Design review of the part built by this model. Coordinates are the model's own, in mm. Face numbers are marked on the shaded views. A direction names the side the tool comes from. Give positions to 0.01 mm unless a question says otherwise; leave off trailing zeros. Order: outer loops, then holes, each group sorted by start corner. A loop starts at its lowest first (then second) coordinate and runs counter-clockwise, first axis right, second up. Notation, with made-up numbers: (13.25, 61.5) - (69.25, 61.5) arc R19 cw to (69.25, 97.5) - close; hole circle Ø5 at (74.5, 26). An arc over 180 degrees is marked (long way). Write each question's results on one line, items separated by ' | '. Start each with the question number.
```python
from build123d import *

# Parameters (mm, degrees)
SKETCH1_R           = 4.15
BOSS_EXTRUDE1_DEPTH = 10
SKETCH4_R           = 11
CUT_EXTRUDE2_DEPTH  = 7.2
CHAMFER1_SIZE       = 1
FILLET2_R           = 25
FILLET3_R           = 2
FILLET4_R           = 2
FILLET5_DEPTH       = 11
FILLET5_2_ANGLE     = 84.965742
FILLET5_3_ANGLE     = 84.965742
SKETCH5_R           = 2.8
CUT_EXTRUDE3_DEPTH  = 58.10630094
CUT_EXTRUDE5_DEPTH  = 4
SKETCH8_R           = 1.5
CUT_EXTRUDE6_DEPTH  = 58.10630094
SKETCH9_R           = 3.5
CUT_EXTRUDE7_DEPTH  = 3.4


with BuildPart() as part:
    # Sketch1 → Boss-Extrude1 (new body)
    with BuildSketch(Plane.XY):
        with BuildLine():
            Line((12.5, 25), (-12.5, 25))
            ThreePointArc((-12.5, 25), (-30.832208454, 17.504408525), (-50.36, 14.2))
            Line((-50.36, 14.2), (-50.36, -14.2))
            ThreePointArc((-50.36, -14.2), (-30.832208454, -17.504408525), (-12.5, -25))
            Line((-12.5, -25), (12.5, -25))
            ThreePointArc((12.5, -25), (37.5, 0), (12.5, 25))
        make_face()
        with Locations((12.5, 0)):
            Circle(SKETCH1_R, mode=Mode.SUBTRACT)
    extrude(amount=BOSS_EXTRUDE1_DEPTH)

    # Sketch4 → Cut-Extrude2 (cut)
    with BuildSketch(Plane.XY.offset(10)):
        with Locations((12.5, 0)):
            Circle(SKETCH4_R)
    extrude(amount=-CUT_EXTRUDE2_DEPTH, mode=Mode.SUBTRACT)

    # Chamfer1
    chamfer1_edges = [part.edges().sort_by_distance(p)[0] for p in [
        (1.5, 0, 10),
    ]]
    chamfer(chamfer1_edges, length=CHAMFER1_SIZE)

    # Fillet2
    fillet2_edges = [part.edges().sort_by_distance(p)[0] for p in [
        (-12.5, 25, 5),
        (-12.5, -25, 5),
    ]]
    fillet(fillet2_edges, radius=FILLET2_R)

    # Fillet3
    fillet3_edges = [part.edges().sort_by_distance(p)[0] for p in [
        (-33.37388042, 16.819399365, 0),
        (2.975273986, -25, 0),
        (-12.003831035, -24.397740667, 0),
        (-12.003831035, 24.397740667, 0),
        (-50.36, 0, 0),
        (2.975273986, 25, 0),
        (37.5, 0, 0),
        (-33.37388042, -16.819399365, 0),
    ]]
    fillet(fillet3_edges, radius=FILLET3_R)

    # Fillet4
    # the kernel refuses this fillet: 2 mm, written as the material it takes off along each edge
    with BuildSketch(Plane(origin=(12.5, 0, 10), x_dir=(0, -1, 0), z_dir=(-1, 0, 0))) as fillet4_piece_1:
        with BuildLine():
            CenterArc((25 - FILLET4_R, -FILLET4_R), FILLET4_R, 0, 90)
            Line((25, -FILLET4_R), (25, 0))
            Line((25, 0), (25 - FILLET4_R, 0))
        make_face()
    revolve(axis=Axis((12.5, 0, 10), (0, 0, 1)), revolution_arc=180, mode=Mode.SUBTRACT)
    with BuildSketch(Plane(origin=(12.5, 25, 10), x_dir=(0, -1, 0), z_dir=(-1, 0, 0))) as fillet4_piece_2:
        with BuildLine():
            CenterArc((FILLET4_R, -FILLET4_R), FILLET4_R, 90, 90)
            Line((0, -FILLET4_R), (0, 0))
            Line((0, 0), (FILLET4_R, 0))
        make_face()
    extrude(amount=34.049452029, mode=Mode.SUBTRACT)
    with BuildSketch(Plane(origin=(-21.549452029, -25, 10), x_dir=(0, 0, -1), z_dir=(1, 0, 0))) as fillet4_piece_3:
        with BuildLine():
            CenterArc((FILLET4_R, FILLET4_R), FILLET4_R, 180, 90)
            Line((0, FILLET4_R), (0, 0))
            Line((0, 0), (FILLET4_R, 0))
        make_face()
    extrude(amount=34.049452029, mode=Mode.SUBTRACT)

    # Fillet5: read off the stored shape, not the designer's step
    # Fillet5 outline → Fillet5 (cut)
    with BuildSketch(Plane.XY):
        with BuildLine():
            Line((-50.36, 14.2), (-50.36, 11.410663893))
            ThreePointArc((-50.36, 11.410663893), (-49.572437829, 13.436773182), (-47.623254098, 14.399091118))
            ThreePointArc((-47.623254098, 14.399091118), (-48.990868253, 14.289114994), (-50.36, 14.2))
        make_face()
        with BuildLine():
            ThreePointArc((-47.623254098, -14.399091118), (-49.572437829, -13.436773182), (-50.36, -11.410663893))
            Line((-50.36, -11.410663893), (-50.36, -14.2))
            ThreePointArc((-50.36, -14.2), (-48.990868253, -14.289114994), (-47.623254098, -14.399091118))
        make_face()
    extrude(amount=FILLET5_DEPTH, mode=Mode.SUBTRACT)

    # Fillet5 2 outline → Fillet5 2 (revolve, cut)
    with BuildSketch(Plane(origin=(-47.36, 11.410663893, 0), x_dir=(-0.08775136609960318, 0.9961424083672241, 0), z_dir=(0.9961424083672241, 0.08775136609960318, 0))):
        with BuildLine():
            ThreePointArc((3, 2), (2.414213562, 0.585786438), (1, 0))
            Line((1, 0), (3, 0))
            Line((3, 0), (3, 2))
        make_face()
    revolve(axis=Axis((-47.36, 11.410663893, 0), (0, 0, 1)), revolution_arc=FILLET5_2_ANGLE, mode=Mode.SUBTRACT)

    # Fillet5 3 outline → Fillet5 3 (revolve, cut)
    with BuildSketch(Plane(origin=(-47.36, -11.410663893, 0), x_dir=(-1, 0, 0), z_dir=(0, 1, 0))):
        with BuildLine():
            ThreePointArc((3, 2), (2.414213562, 0.585786438), (1, 0))
            Line((1, 0), (3, 0))
            Line((3, 0), (3, 2))
        make_face()
    revolve(axis=Axis((-47.36, -11.410663893, 0), (0, 0, 1)), revolution_arc=FILLET5_3_ANGLE, mode=Mode.SUBTRACT)

    # Sketch5 → Cut-Extrude3 (cut, through all)
    with BuildSketch(Plane(origin=(0, 0, 0), x_dir=(-1, 0, 0), z_dir=(0, 0, -1))):
        with Locations((40.16, 0)):
            Circle(SKETCH5_R)
    extrude(amount=-CUT_EXTRUDE3_DEPTH, mode=Mode.SUBTRACT)

    # Sketch7 → Cut-Extrude5 (cut)
    with BuildSketch(Plane(origin=(0, 0, 0), x_dir=(-1, 0, 0), z_dir=(0, 0, -1))):
        Polygon((36.16, -2.309401077), (40.16, -4.618802154), (44.16, -2.309401077), (44.16, 2.309401077), (40.16, 4.618802154), (36.16, 2.309401077), align=None)
    extrude(amount=-CUT_EXTRUDE5_DEPTH, mode=Mode.SUBTRACT)

    # Sketch8 → Cut-Extrude6 (cut, through all)
    with BuildSketch(Plane(origin=(0, 0, 0), x_dir=(-1, 0, 0), z_dir=(0, 0, -1))):
        with Locations((43.36, -8.5)):
            Circle(SKETCH8_R)
        with Locations((28.36, -8.5)):
            Circle(SKETCH8_R)
        with Locations(Location((28.36, 8.5, 0), (0, 0, 180))):
            Circle(SKETCH8_R)
        with Locations(Location((43.36, 8.5, 0), (0, 0, 180))):
            Circle(SKETCH8_R)
    extrude(amount=-CUT_EXTRUDE6_DEPTH, mode=Mode.SUBTRACT)

    # Sketch9 → Cut-Extrude7 (cut)
    with BuildSketch(Plane(origin=(0, 0, 0), x_dir=(-1, 0, 0), z_dir=(0, 0, -1))):
        with Locations((43.36, -8.5)):
            Circle(SKETCH9_R)
        with Locations((28.36, -8.5)):
            Circle(SKETCH9_R)
        with Locations(Location((28.36, 8.5, 0), (0, 0, 180))):
            Circle(SKETCH9_R)
        with Locations(Location((43.36, 8.5, 0), (0, 0, 180))):
            Circle(SKETCH9_R)
    extrude(amount=-CUT_EXTRUDE7_DEPTH, mode=Mode.SUBTRACT)


solid = part.part
```
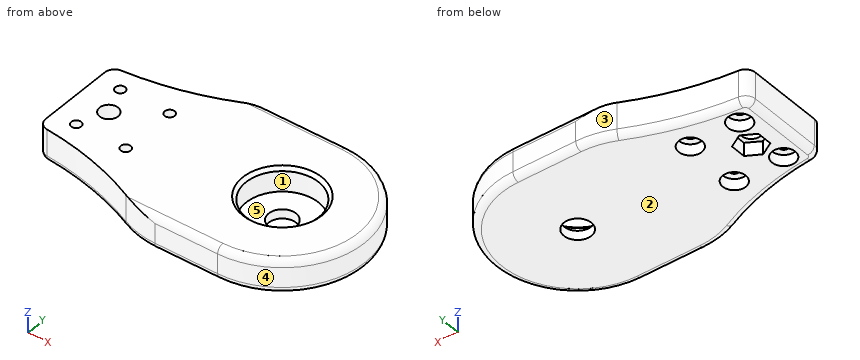
Q1. Insertion check: pin 1 Ø3.5 at (x, y) = (-43.36, 8.5) entering from -Z; pin 2 Ø4 at (x, z) = (-29, 6) entering from +Y; pin 3 Ø2 at (x, z) = (23.5, 6) entering from +Y. Each pin has a flat end and moves straight along its axis. Give the tip position at first contact, or say it passes through.
Q2. Add section A-A (y = 0). Give the boundary of the cut face in (x, z), plus the area to 3 significant figures.
Q3. Add section B-B (z = 5.5). Give the boundary of the cut face in (x, y), plus the area to 3 significant figures.
Q4. Add section C-C (x = -28.36). Give the number of separate pieces and of enclosed holes in the cut face, plus the area to 3 significant figures.
Q5. Machinability: for the marked faces 4 and 5, which of the approach directions +Z, -Z, +X, -X, +Y, -Y give a long, thin tool a straight path to every point of the face, cutting with its end or side? Answer none if there is none.
Q6. Draft analysis for pull direction X (two halves, no side actions). For the marked faces 1, 2 and 3, state which applies: pulls with the +X half, pulls with the -X half, needs draft (parallel to the pull), parting line crosses it, or undercut.
Q7. For line 1 (X direction, y = 0, z = 2.2); line 2 (X direction, y = -1, z = 6); line 3 (Y direction, x = -28.36, z = 0.75), list the stretches that pass through material, from the lowest coordinate up. Write a range as [from, to].
Verdict:
1) pin 1: stops at z = 3.4 | pin 2: stops at y = 18.69 | pin 3: stops at y = 22.91
2) outline: (-50.36, 2) arc R2 ccw to (-48.36, 0) - (-44.16, 0) - (-44.16, 4) - (-42.96, 4) - (-42.96, 10) - (-50.36, 10) - close; (-37.36, 4) - (-36.16, 4) - (-36.16, 0) - (8.35, 0) - (8.35, 2.8) - (1.5, 2.8) - (1.5, 9) - (0.5, 10) - (-37.36, 10) - close; (16.65, 0) - (35.5, 0) arc R2 ccw to (37.5, 2) - (37.5, 8) arc R2 ccw to (35.5, 10) - (24.5, 10) - (23.5, 9) - (23.5, 2.8) - (16.65, 2.8) - close | area: 628 mm2
3) outline: (-50.36, -11.41) arc R3 ccw to (-47.62, -14.4) arc R90 cw to (-17.2, -22.62) arc R25 ccw to (-6.55, -25) - (12.5, -25) arc R25 ccw to (12.5, 25) - (-6.55, 25) arc R25 ccw to (-17.2, 22.62) arc R90 cw to (-47.62, 14.4) arc R3 ccw to (-50.36, 11.41) - close; hole circle Ø3 at (-43.36, -8.5); hole circle Ø3 at (-43.36, 8.5); hole circle Ø5.6 at (-40.16, 0); hole circle Ø3 at (-28.36, -8.5); hole circle Ø3 at (-28.36, 8.5); hole circle Ø22 at (12.5, 0) | area: 3,160 mm2
4) separate pieces: 3 | enclosed holes: 0 | area: 276 mm2
5) face 4: +Z, -Z, +X | face 5: +Z
6) face 1: undercut | face 2: needs draft | face 3: pulls with the -X half
7) line 1: x = [-50.36, -44.16], [-36.16, 8.35], [16.65, 37.5] | line 2: x = [-50.36, -42.78], [-37.54, 1.55], [23.45, 37.48] | line 3: y = [-17.79, -12], [-5, 5], [12, 17.79]
